Verification items for the finished model (mm, model axes). A direction names the side the tool comes from. Give positions to 0.01 mm unless a question says otherwise; leave off trailing zeros. Write each loop counter-clockwise with the first axis right and the second up, starting at its lowest first coordinate (ties: lowest second). Pieces come first, ordered by that corner, then holes.
from build123d import *

# Parameters (mm, degrees)
F0_W     = 12.5
F0_H     = 24
F1_DEPTH = 6
F0_W_2   = 20
F0_H_2   = 108
F0_R     = 1.5
F0_W_3   = 6
F2_DEPTH = 26
F5_DEPTH = 30
F6_R     = 2.99999


# Not quite as in the source:
# - a fillet or chamfer is up to 0.001 mm smaller than in the source, because OpenCascade refuses the exact size


with BuildPart() as f1:
    # F0 (on Top) → F1 (new body)
    with BuildSketch(Plane.XY):
        with Locations((6.25, -36)):
            Rectangle(F0_W, F0_H)
    extrude(amount=F1_DEPTH)



with BuildPart() as f1b:
    # F0 (on Top) → F1, piece 2 (new body)
    with BuildSketch(Plane.XY):
        Polygon((11.0289425277, -20), (0, -9.1190332702), (0, -20), align=None)
    extrude(amount=F1_DEPTH)


with BuildPart() as f1c:
    # F0 (on Top) → F1, piece 3 (new body)
    with BuildSketch(Plane.XY):
        with Locations((6.25, 36)):
            Rectangle(F0_W, F0_H)
    extrude(amount=F1_DEPTH)


with BuildPart() as f1d:
    # F0 (on Top) → F1, piece 4 (new body)
    with BuildSketch(Plane.XY):
        with Locations((-18, 0)):
            Rectangle(F0_W_2, F0_H_2)
        with Locations((-22, -40)):
            Circle(F0_R, mode=Mode.SUBTRACT)
        with Locations((-14, -40)):
            Circle(F0_R, mode=Mode.SUBTRACT)
        with Locations((-22, -20)):
            Circle(F0_R, mode=Mode.SUBTRACT)
        with Locations((-14, -20)):
            Circle(F0_R, mode=Mode.SUBTRACT)
        with Locations((-22, 0)):
            Circle(F0_R, mode=Mode.SUBTRACT)
        with Locations((-22, 20)):
            Circle(F0_R, mode=Mode.SUBTRACT)
        with Locations((-14, 0)):
            Circle(F0_R, mode=Mode.SUBTRACT)
        with Locations((-14, 20)):
            Circle(F0_R, mode=Mode.SUBTRACT)
        with Locations((-22, 40)):
            Circle(F0_R, mode=Mode.SUBTRACT)
        with Locations((-14, 40)):
            Circle(F0_R, mode=Mode.SUBTRACT)
    extrude(amount=F1_DEPTH)


with BuildPart() as f1e:
    # F0 (on Top) → F1, piece 5 (new body)
    with BuildSketch(Plane.XY):
        Polygon((0, 20), (0, 9.1568542495), (10.8431457505, 20), align=None)
    extrude(amount=F1_DEPTH)


with BuildPart() as f1_1:
    add(f1.part)

    add(f1b.part)  # F2 merges F1b

    add(f1c.part)  # F2 merges F1c

    add(f1d.part)  # F2 merges F1d

    add(f1e.part)  # F2 merges F1e
    # F0 (on Top) → F2 (join)
    with BuildSketch(Plane.XY):
        Polygon((18.5, 22), (18.5, 48), (31.5, 48), (31.5, 22), (37.5, 22), (37.5, 54), (-8, 54), (-8, -54), (37.5, -54), (37.5, -22), (31.5, -22), (31.5, -48), (18.5, -48), (18.5, -21.7517847015), (0, -3.5), (0, 3.5), align=None)
        with Locations((6.25, -36)):
            Rectangle(F0_W, F0_H, mode=Mode.SUBTRACT)
        Polygon((0, -20), (0, -9.1190332702), (11.0289425277, -20), align=None, mode=Mode.SUBTRACT)
        Polygon((10.8431457505, 20), (0, 9.1568542495), (0, 20), align=None, mode=Mode.SUBTRACT)
        with Locations((6.25, 36)):
            Rectangle(F0_W, F0_H, mode=Mode.SUBTRACT)
        with Locations((-31, 0)):
            Rectangle(F0_W_3, F0_H_2)
    extrude(amount=F2_DEPTH)

    # F4 (on offset) → F5 (cut)
    with BuildSketch(Plane.YZ.offset(37.5)):
        with BuildLine():
            ThreePointArc((-34, 18.5), (-36.5, 16), (-34, 13.5))
            Line((-34, 13.5), (-30, 13.5))
            ThreePointArc((-30, 13.5), (-27.5, 16), (-30, 18.5))
            Line((-30, 18.5), (-34, 18.5))
        make_face()
        with BuildLine():
            Line((34, 18.5), (30, 18.5))
            ThreePointArc((30, 18.5), (27.5, 16), (30, 13.5))
            Line((30, 13.5), (34, 13.5))
            ThreePointArc((34, 13.5), (36.5, 16), (34, 18.5))
        make_face()
    extrude(amount=-F5_DEPTH, mode=Mode.SUBTRACT)

    # F6 (radius 3 in the source; OpenCascade refuses exactly that, so slightly less here)
    f6_edges = [f1_1.edges().sort_by_distance(p)[0] for p in [
        (0, 48, 16),
        (18.5, 48, 13),
        (31.5, 48, 13),
        (12.5, 48, 16),
        (12.5, -24, 16),
        (0, -24, 16),
        (0, 20, 16),
        (0, -9.119033, 16),
        (0, -20, 16),
        (11.028943, -20, 16),
        (10.843146, 20, 16),
        (0, 9.156854, 16),
        (0, -48, 16),
        (18.5, -48, 13),
        (0, 24, 16),
        (12.5, 24, 16),
        (12.5, -48, 16),
        (31.5, -48, 13),
        (37.5, -54, 13),
        (37.5, 54, 13),
        (34.5, 22, 26),
        (34.5, -22, 26),
        (34.5, -22, 0),
        (34.5, 22, 0),
        (0, -3.5, 13),
        (0, 3.5, 13),
        (18.5, -21.751785, 13),
        (18.5, 22, 13),
        (31.5, 22, 13),
        (37.5, 22, 13),
        (31.5, -22, 13),
        (37.5, -22, 13),
        (-31, -54, 26),
        (-31, 54, 26),
        (-34, 0, 0),
        (-28, 0, 26),
        (-8, 0, 26),
        (-34, 0, 26),
    ]]
    fillet(f6_edges, radius=F6_R)


solid = f1_1.part
Item 1: Set-up check for faces 5 (the face through (18.5, 34, 13)), 6 (the face through (36.64, -22.9, 13.18)), 7 (the face through (34.5, -36.5, 16.1)), 8 (the face through (6, 48, 16)), 9 (the face through (34.54, 23.31, 25.48)): record each of +Z, -Z, +X, -X, +Y, -Y from which the full face is reachable in a straight line by a thin tool's end or side.
Answer key:
face 5: +Z, -Z
face 6: +Z, -Z, +X
face 7: +X
face 8: +Z
face 9: +Z, +X
Item 2: Sectioned sample at B-B on y = 32. State how many separate pieces and enclosed holes the cut face has, then the cut area to 3 significant figures.
Answer key:
separate pieces: 4
enclosed holes: 0
area: 803 mm2
Item 3: Release check for a two-part mould opening along X. For faces 1 (the face through (-7.1, -0.76, 25.14)), 2 (the face through (-8, 1, 14)), 3 (the face through (-30.96, -53.48, 24.69)), 4 (the face through (0, 0, 13)) record: released by +X, released by -X, zero draft, split by the parting line, or undercut.
Answer key:
face 1: undercut
face 2: undercut
face 3: zero draft
face 4: released by +X
Item 4: Sectioned sample at A-A on x = -22. Record the cut outline in (y, z).
Answer key:
outline: (-54, 0) - (-41.5, 0) - (-41.5, 6) - (-54, 6) - close; (-38.5, 0) - (-21.5, 0) - (-21.5, 6) - (-38.5, 6) - close; (-18.5, 0) - (-1.5, 0) - (-1.5, 6) - (-18.5, 6) - close; (1.5, 0) - (18.5, 0) - (18.5, 6) - (1.5, 6) - close; (21.5, 0) - (38.5, 0) - (38.5, 6) - (21.5, 6) - close; (41.5, 0) - (54, 0) - (54, 6) - (41.5, 6) - close
Item 5: Depth check by flat-ended pin: pin 1 (1.5 mm diameter, centred on x = -15, y = -39.5, fed in from +Z); pin 2 (5 mm diameter, centred on y = -14.5, z = 12, fed in from +X). Enter the tip coordinate at first touch or a pass-through.
Answer key:
pin 1: stops at z = 6
pin 2: stops at x = 13.68
Item 6: Scan lines: line 1 along X through (y, z) = (39.5, 13.5); line 2 along Y through (x, z) = (-14, 4.2); line 3 along X through (y, z) = (-14.5, 8.25). Record each from-to range of solid material in increasing order.
Answer key:
line 1: x = -34 to -28, -8 to 0, 12.5 to 18.5, 31.5 to 37.5
line 2: y = -54 to -41.5, -38.5 to -21.5, -18.5 to -1.5, 1.5 to 18.5, 21.5 to 38.5, 41.5 to 54
line 3: x = -34 to -28, -8 to 0.59, 5.45 to 11.15
